from build123d import *

# Parameters (mm, degrees)
SKETCH1_W           = 152.4
SKETCH1_H           = 50.8
BOSS_EXTRUDE1_DEPTH = 3.048
SKETCH2_W           = 6.35
SKETCH2_H           = 3.048
CUT_EXTRUDE1_DEPTH  = 81.379663498
SKETCH4_R           = 1.25
SKETCH4_R_2         = 5.08
CUT_EXTRUDE2_DEPTH  = 81.379663498


with BuildPart() as part:
    # Sketch1 → Boss-Extrude1 (new body)
    with BuildSketch(Plane(origin=(0, 0, 0), x_dir=(1, 0, 0), z_dir=(0, 1, 0))):
        Rectangle(SKETCH1_W, SKETCH1_H)
    extrude(amount=BOSS_EXTRUDE1_DEPTH)

    # Sketch2 → Cut-Extrude1 (cut, through all)
    with BuildSketch(Plane(origin=(0, 3.048, 0), x_dir=(1, 0, 0), z_dir=(0, 1, 0))):
        with Locations((-73.025, 23.876)):
            Rectangle(SKETCH2_W, SKETCH2_H)
        with Locations((-60.325, 23.876)):
            Rectangle(SKETCH2_W, SKETCH2_H)
        with Locations((-47.625, 23.876)):
            Rectangle(SKETCH2_W, SKETCH2_H)
        with Locations((-34.925, 23.876)):
            Rectangle(SKETCH2_W, SKETCH2_H)
        with Locations((-22.225, 23.876)):
            Rectangle(SKETCH2_W, SKETCH2_H)
        with Locations((-9.525, 23.876)):
            Rectangle(SKETCH2_W, SKETCH2_H)
        with Locations((15.875, 23.876)):
            Rectangle(SKETCH2_W, SKETCH2_H)
        with Locations((3.175, 23.876)):
            Rectangle(SKETCH2_W, SKETCH2_H)
        with Locations((28.575, 23.876)):
            Rectangle(SKETCH2_W, SKETCH2_H)
        with Locations((41.275, 23.876)):
            Rectangle(SKETCH2_W, SKETCH2_H)
        with Locations((53.975, 23.876)):
            Rectangle(SKETCH2_W, SKETCH2_H)
        with Locations((66.675, 23.876)):
            Rectangle(SKETCH2_W, SKETCH2_H)
        with Locations((-73.025, -23.876)):
            Rectangle(SKETCH2_W, SKETCH2_H)
        with Locations((-60.325, -23.876)):
            Rectangle(SKETCH2_W, SKETCH2_H)
        with Locations((-47.625, -23.876)):
            Rectangle(SKETCH2_W, SKETCH2_H)
        with Locations((-34.925, -23.876)):
            Rectangle(SKETCH2_W, SKETCH2_H)
        with Locations((-22.225, -23.876)):
            Rectangle(SKETCH2_W, SKETCH2_H)
        with Locations((-9.525, -23.876)):
            Rectangle(SKETCH2_W, SKETCH2_H)
        with Locations((3.175, -23.876)):
            Rectangle(SKETCH2_W, SKETCH2_H)
        with Locations((15.875, -23.876)):
            Rectangle(SKETCH2_W, SKETCH2_H)
        with Locations((28.575, -23.876)):
            Rectangle(SKETCH2_W, SKETCH2_H)
        with Locations((41.275, -23.876)):
            Rectangle(SKETCH2_W, SKETCH2_H)
        with Locations((53.975, -23.876)):
            Rectangle(SKETCH2_W, SKETCH2_H)
        with Locations((66.675, -23.876)):
            Rectangle(SKETCH2_W, SKETCH2_H)
    extrude(amount=-CUT_EXTRUDE1_DEPTH, mode=Mode.SUBTRACT)

    # Sketch4 → Cut-Extrude2 (cut, through all)
    with BuildSketch(Plane(origin=(0, 3.048, 0), x_dir=(1, 0, 0), z_dir=(0, 1, 0))):
        with Locations(Location((-61.89, -5.08, 0), (0, 0, 270))):
            Circle(SKETCH4_R)
        with Locations(Location((-44.79, -5.08, 0), (0, 0, 270))):
            Circle(SKETCH4_R)
        with Locations(Location((-53.34, -5.08, 0), (0, 0, 270))):
            Circle(SKETCH4_R_2)
        with Locations(Location((44.79, -5.08, 0), (0, 0, 270))):
            Circle(SKETCH4_R)
        with Locations(Location((53.34, -5.08, 0), (0, 0, 270))):
            Circle(SKETCH4_R_2)
        with Locations(Location((61.89, -5.08, 0), (0, 0, 270))):
            Circle(SKETCH4_R)
    extrude(amount=-CUT_EXTRUDE2_DEPTH, mode=Mode.SUBTRACT)


solid = part.part
Geometry check sheet. Reference: the model listing, model coordinates, mm. A direction names the side the tool comes from. Round coordinates to 2 decimals unless told otherwise and drop trailing zeros. Write each loop counter-clockwise with the first axis right and the second up, starting at its lowest first coordinate (ties: lowest second). Pieces come first, ordered by that corner, then holes. Notation, with made-up numbers: (72, 17) - (130, 17) arc R20 ccw to (130, 55) - close; hole circle Ø7 at (77.5, 70.5). An arc over 180 degrees is marked (long way). One line per item, written item: value.
1. Cross-section at B-B on y = 0.5. Give the number of separate pieces and of enclosed holes in the cut face, and give its area (3 significant figures).
The answers:
separate pieces: 1
enclosed holes: 6
area: 7,100 mm^2
2. Set-up check for faces 4 (the face through (-19.05, 2, -24)), 5 (the face through (-12.7, 2, 24)), 6 (the face through (-76.2, 2, 0)), 7 (the face through (-69.85, 2, 24)), 8 (the face through (-57.85, 1.55, 7.42)): record each of +Z, -Z, +X, -X, +Y, -Y from which the full face is reachable in a straight line by a thin tool's end or side.
The answers:
face 4: -Z, +Y, -Y
face 5: +Z, +Y, -Y
face 6: +Z, -Z, -X, +Y, -Y
face 7: +Z, -X, +Y, -Y
face 8: +Y, -Y
3. Depth check by flat-ended pin: pin 1 Ø1.5 at (y, z) = (1.5, -23.5) entering from -X; pin 2 Ø2 at (x, z) = (61.89, 5.08) entering from +Y; pin 3 Ø0.9 at (x, y) = (67, 1.5) entering from +Z. Enter the tip coordinate at first touch or a pass-through.
The answers:
pin 1: stops at x = -69.85
pin 2: passes through
pin 3: stops at z = 22.35
4. Cross-section at A-A on x = -53.34. Record the boundary of the cut face in (y, z).
The answers:
outline: (0, -25.4) - (3.05, -25.4) - (3.05, 0) - (0, 0) - close; (0, 10.16) - (3.05, 10.16) - (3.05, 25.4) - (0, 25.4) - close
5. Mould release check, pull along Z, two halves, no side actions. Record for faces 1 (the face through (76.2, 2, 0)), 2 (the face through (63.13, 1.55, 4.92)), 3 (the face through (-67, 2, 25.4)): released by +Z, released by -Z, zero draft, split by the parting line, or undercut.
The answers:
face 1: zero draft
face 2: undercut
face 3: released by +Z
6. Scan lines: L1, parallel to X at y = 1.65, z = 9; L2, parallel to Z at x = -34, y = 1.6; L3, parallel to Z at x = -55, y = 2.2. Record each from-to range of solid material in increasing order.
The answers:
L1: x = -76.2 to -56.57, -50.11 to 50.11, 56.57 to 76.2
L2: z = -22.35 to 22.35
L3: z = -25.4 to 0.28, 9.88 to 25.4
